```python
from build123d import *

# Parameters (mm, degrees)
CORTE_EXTERIOR_R        = 3.500002593
SALIENTE_EXTRUIR1_DEPTH = 3
CORTAR_EXTRUIR1_DEPTH   = 1
CORTAR_EXTRUIR2_DEPTH   = 0.1


with BuildPart() as part:
    # Corte exterior → Saliente-Extruir1 (new body)
    with BuildSketch(Plane.XY):
        with BuildLine():
            Line((47.504320945, 38.211786495), (51.847305041, 38.211786495))
            ThreePointArc((51.847305041, 38.211786495), (55.534254627, 41.572373104), (54.480090972, 46.448424641))
            ThreePointArc((54.480090972, 46.448424641), (30.004320476, 57.31391234), (5.528550918, 46.448424641))
            ThreePointArc((5.528550918, 46.448424641), (4.474387263, 41.572373104), (8.161336848, 38.211786495))
            Line((8.161336848, 38.211786495), (12.511035037, 38.211786495))
            ThreePointArc((12.511035037, 38.211786495), (15.339462162, 37.04021362), (16.511035037, 34.211786495))
            Line((16.511035037, 34.211786495), (16.504320945, -26.686088981))
            ThreePointArc((16.504320945, -26.686088981), (17.67589382, -29.514516106), (20.504320945, -30.686088981))
            Line((20.504320945, -30.686088981), (39.504320945, -30.686088981))
            ThreePointArc((39.504320945, -30.686088981), (42.33274807, -29.514516106), (43.504320945, -26.686088981))
            Line((43.504320945, -26.686088981), (43.504320945, 34.211786495))
            ThreePointArc((43.504320945, 34.211786495), (44.67589382, 37.04021362), (47.504320945, 38.211786495))
        make_face()
        with Locations((30.00431952, 24.313911283)):
            Circle(CORTE_EXTERIOR_R, mode=Mode.SUBTRACT)
        with BuildLine():
            ThreePointArc((52.277272453, 44.456319148), (30.004320476, 54.343913397), (7.731367869, 44.456320565))
            Line((7.731367869, 44.456320565), (10.253113799, 42.175794866))
            ThreePointArc((10.253113799, 42.175794866), (30.004320476, 50.943913397), (49.755526523, 42.175793449))
            Line((49.755526523, 42.175793449), (52.277272453, 44.456319148))
        make_face(mode=Mode.SUBTRACT)
    extrude(amount=SALIENTE_EXTRUIR1_DEPTH)

    # Grabado Superficie → Cortar-Extruir1 (cut)
    with BuildSketch(Plane.XY):
        with BuildLine():
            Line((32.873672963, 22.309708905), (31.999357171, 9.92309063))
            ThreePointArc((31.999357171, 9.92309063), (30.004320945, 8.063911283), (28.009284719, 9.92309063))
            Line((28.009284719, 9.92309063), (27.134968927, 22.309708905))
            ThreePointArc((27.134968927, 22.309708905), (30.004320945, 20.813910115), (32.873672963, 22.309708905))
        make_face()
    extrude(amount=CORTAR_EXTRUIR1_DEPTH, mode=Mode.SUBTRACT)

    # grabado linea medio → Cortar-Extruir2 (cut)
    with BuildSketch(Plane.XY):
        Polygon((16.504320945, -26.046088981), (24.644320945, -26.046088981), (24.644320945, -30.686088981), (27.164320945, -30.686088981), (27.164320945, -26.044872481), (43.504320945, -25.844872481), (43.504320945, -2.816088981), (27.164320945, -2.816088981), (27.164320945, 1.823911019), (24.644320945, 1.823911019), (24.644320945, -2.816088981), (20.584320945, -2.816088981), (20.584320945, -10.896088981), (16.504320945, -10.896088981), align=None)
    extrude(amount=CORTAR_EXTRUIR2_DEPTH, mode=Mode.SUBTRACT)


solid = part.part
```
Geometry check sheet. Reference: the model listing, model coordinates, mm. A direction names the side the tool comes from. Coordinates: 2 decimals unless noted, no trailing zeros. Write each loop counter-clockwise with the first axis right and the second up, starting at its lowest first coordinate (ties: lowest second). Pieces come first, ordered by that corner, then holes. Notation, with made-up numbers: (58.25, 74.5) -> (99.25, 74.5) arc R18 ccw to (99.25, 99.5) -> close; hole circle Ø6 at (27.25, -5.5). An arc over 180 degrees is marked (long way). Use CSV: the item, a comma, the result in double quotes. Start each with the question number.
Item 1: Cross-section at B-B, the plane z = 2.25. Record the cut outline in (x, y).
Item 2: Cross-section at C-C, the plane x = 23.5. Record the cut outline in (y, z).
Item 3: Mould release check, pull along X, two halves, no side actions. Record for faces 4 (the cylindrical face through (30.046, 8.064, 0.493)), 5 (the cylindrical face through (17.64, -29.48, 1.48)), 6 (the flat face through (30, 15, 1)), 7 (the cylindrical face through (55.51, 41.5, 1.48)): released by +X, released by -X, zero draft, split by the parting line, or undercut.
Item 4: Depth check by flat-ended pin: pin 1 Ø0.9 at (y, z) = (-2, 2) entering from -X; pin 2 Ø0.9 at (y, z) = (-9.5, 2) entering from +X; pin 3 Ø4.5 at (x, y) = (31, 14.5) entering from -Z. Enter the tip coordinate at first touch or a pass-through.
Item 5: Cross-section at D-D, the plane y = 0.5. Record the cut outline in (x, z), plus the area to 3 significant figures.
Item 6: Set-up check for faces 1 (the flat face through (30, -30.686, 1)), 2 (the flat face through (43.504, 3, 1)), 3 (the flat face through (51, 43.3, 1.5)): record each of +Z, -Z, +X, -X, +Y, -Y from which the full face is reachable in a straight line by a thin tool's end or side.
Item 7: Cross-section at A-A, the plane x = 31. Record the cut outline in (y, z), plus the area to 3 significant figures.
Item 8: Thickness scan on line 1 (X direction, y = 46, z = 0.6); line 2 (Z direction, x = 37, y = -15.5); line 3 (X direction, y = -15, z = 0.55). Record the ranges inside material, lowest first.
Answers:
1,outline,"(5.53, 46.45) arc R5 ccw to (8.16, 38.21) -> (12.51, 38.21) arc R4 cw to (16.51, 34.21) -> (16.5, -26.69) arc R4 ccw to (20.5, -30.69) -> (39.5, -30.69) arc R4 ccw to (43.5, -26.69) -> (43.5, 34.21) arc R4 cw to (47.5, 38.21) -> (51.85, 38.21) arc R5 ccw to (54.48, 46.45) arc R33 ccw to start; hole (7.73, 44.46) -> (10.25, 42.18) arc R26.63 cw to (49.76, 42.18) -> (52.28, 44.46) arc R30.03 ccw to start; hole circle Ø7 at (30, 24.31)"
2,outline,"(-30.69, 0) -> (-26.05, 0) -> (-26.05, 0.1) -> (-2.82, 0.1) -> (-2.82, 0) -> (50.14, 0) -> (50.14, 3) -> (-30.69, 3) -> close; (53.63, 0) -> (56.67, 0) -> (56.67, 3) -> (53.63, 3) -> close"
3,face 4,"undercut"
3,face 5,"released by -X"
3,face 6,"undercut"
3,face 7,"released by +X"
4,pin 1,"x = 16.51"
4,pin 2,"x = 43.5"
4,pin 3,"z = 0"
5,outline,"(16.51, 0) -> (24.64, 0) -> (24.64, 0.1) -> (27.16, 0.1) -> (27.16, 0) -> (43.5, 0) -> (43.5, 3) -> (16.51, 3) -> close"
5,area,"80.7 mm^2"
6,face 1,"+Z, -Z, +X, -X, -Y"
6,face 2,"+Z, -Z, +X, -Y"
6,face 3,"+Z, -Z"
7,outline,"(-30.69, 0) -> (-26, 0) -> (-26, 0.1) -> (-2.82, 0.1) -> (-2.82, 0) -> (8.33, 0) -> (8.33, 1) -> (20.96, 1) -> (20.96, 3) -> (-30.69, 3) -> close; (27.67, 0) -> (50.93, 0) -> (50.93, 3) -> (27.67, 3) -> close; (54.33, 0) -> (57.3, 0) -> (57.3, 3) -> (54.33, 3) -> close"
7,area,"219 mm^2"
8,line 1,"5.17 to 9.23, 14.55 to 45.46, 50.78 to 54.84"
8,line 2,"0.1 to 3"
8,line 3,"16.51 to 43.5"
